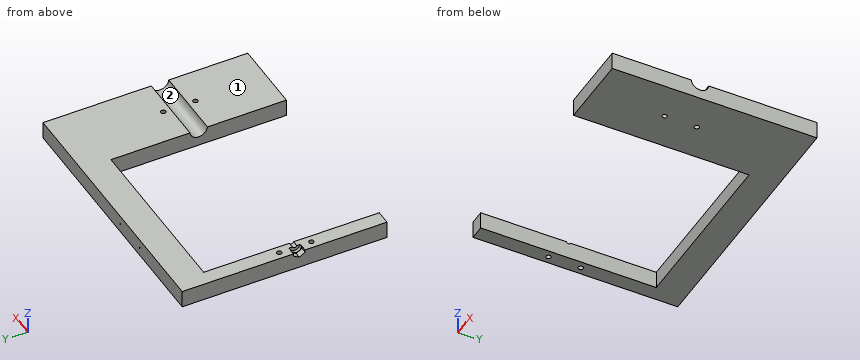
```python
from build123d import *

# Parameters (mm, degrees)
F0_W      = 180
F0_H      = 140
F1_DEPTH  = 30
F4_DEPTH  = 30
F5_DEPTH  = 4
F6_R      = 3.8
F7_DEPTH  = 2
F8_R      = 1.55
F9_DEPTH  = 7
F10_R     = 6
F12_DEPTH = 50
F11_R     = 0.5
F13_DEPTH = 1
F14_W     = 180
F14_H     = 140
F15_DEPTH = 18
F16_R     = 1.65
F17_DEPTH = 12


# Not quite as in the source:
# - a feature names something its author has since deleted; it is built from what else it names


with BuildPart() as f1:
    # F0 (on Top) → F1 (new body)
    with BuildSketch(Plane.XY):
        Rectangle(F0_W, F0_H)
    extrude(amount=F1_DEPTH)

    # F3 (on Top) → F4 (cut, through all)
    with BuildSketch(Plane.XY):
        Polygon((40, -70), (40, 0), (40, 50), (0, 50), (-80, 50), (-80, -70), align=None)
    extrude(amount=F4_DEPTH, mode=Mode.SUBTRACT)

    # F2 (on face) → F5 (cut)
    with BuildSketch(Plane(origin=(-90, 0, 0), x_dir=(0, -1, 0), z_dir=(-1, 0, 0))):
        Polygon((10, 17.12), (5.9989626345, 14.81), (5.9989626345, 10.19), (10, 7.88), (14.0010373655, 10.19), (14.0010373655, 14.81), align=None)
    extrude(amount=-F5_DEPTH, mode=Mode.SUBTRACT)

    # F6 (on face) → F7 (cut)
    with BuildSketch(Plane(origin=(-86, 0, 0), x_dir=(0, -1, 0), z_dir=(-1, 0, 0))):
        with Locations((10, 12.5)):
            Circle(F6_R)
    extrude(amount=-F7_DEPTH, mode=Mode.SUBTRACT)

    # F8 (on face) → F9 (cut)
    with BuildSketch(Plane(origin=(-84, 0, 0), x_dir=(0, -1, 0), z_dir=(-1, 0, 0))):
        with Locations((10, 12.5)):
            Circle(F8_R)
    extrude(amount=-F9_DEPTH, mode=Mode.SUBTRACT)

    # F10 (on face) → F12 (cut, through all)
    with BuildSketch(Plane.YZ.offset(90)):
        with Locations((-10, 12.5)):
            Circle(F10_R)
    extrude(amount=-F12_DEPTH, mode=Mode.SUBTRACT)

    # F11 (on face) → F13 (cut)
    with BuildSketch(Plane(origin=(0, 70, 0), x_dir=(-1, 0, 0), z_dir=(0, 1, 0))):
        with Locations((35, 6)):
            Circle(F11_R)
        with Locations((10, 6)):
            Circle(F11_R)
    extrude(amount=-F13_DEPTH, mode=Mode.SUBTRACT)

    # F14 (on face) → F15 (cut)
    with BuildSketch(Plane.XY.offset(30)):
        Rectangle(F14_W, F14_H)
    extrude(amount=-F15_DEPTH, mode=Mode.SUBTRACT)

    # F16 (on face) → F17 (cut, through all)
    with BuildSketch(Plane.XY.offset(12)):
        with Locations((65, 1)):
            Circle(F16_R)
        with Locations((65, -21)):
            Circle(F16_R)
        with Locations((-85, 1)):
            Circle(F16_R)
        with Locations((-85, -21)):
            Circle(F16_R)
    extrude(amount=-F17_DEPTH, mode=Mode.SUBTRACT)


solid = f1.part
```
Verification items for the finished model (mm, model axes). Face numbers are marked on the shaded views. Coordinates: 2 decimals unless noted, no trailing zeros. Write each loop counter-clockwise with the first axis right and the second up, starting at its lowest first coordinate (ties: lowest second). Pieces come first, ordered by that corner, then holes. Notation, with made-up numbers: (33, -1) - (45, -1) arc R20 cw to (45, 10) - close; hole circle Ø7 at (-4, 21.25). An arc over 180 degrees is marked (long way). Write item = value, one per line.
Q1. Cross-section at A-A (y = -56.5). Enter the section's corners in (x, z), plus the area to 3 significant figures.
Answer:
outline = (-90, 0) - (-80, 0) - (-80, 12) - (-90, 12) - close; (40, 0) - (90, 0) - (90, 12) - (40, 12) - close
area = 720 mm²
Q2. Mould release check, pull along Y, two halves, no side actions. Record for the marked faces 1 and 2: released by +Y, released by -Y, zero draft, split by the parting line, or undercut.
Answer:
face_1 = zero draft
face_2 = undercut
Q3. Cross-section at B-B (z = 2). Enter the section's corners in (x, y).
Answer:
outline = (-90, -70) - (-80, -70) - (-80, 50) - (40, 50) - (40, -70) - (90, -70) - (90, 70) - (-90, 70) - close; hole circle Ø3.3 at (-85, -21); hole circle Ø3.3 at (-85, 1); hole circle Ø3.3 at (65, -21); hole circle Ø3.3 at (65, 1)
Q4. Material ranges on L1, parallel to Y at x = 65, z = 5.75; L2, parallel to Z at x = -35, y = 69.4; L3, parallel to X at y = -17, z = 5, recorded low to high. Write a range as from..to.
Answer:
L1 = -70..-22.65, -19.35..-0.65, 2.65..70
L2 = 0..5.5, 6.5..12
L3 = -90..-80, 40..90
Q5. Go/stop test with flat-tipped pins: pin 1 Ø4.5 at (x, y) = (65, -21) entering from +Z; pin 2 Ø2.5 at (x, y) = (-85, -21) entering from -Z; pin 3 Ø3 at (x, z) = (-26.5, 3) entering from -Y; pin 4 Ø1.2 at (y, z) = (-10.5, 9) entering from -X. Record where each tip stops, or that it passes through.
Answer:
pin_1 = 12
pin_2 = through
pin_3 = 50
pin_4 = -86
Q6. Cross-section at C-C (x = 28). Enter the section's corners in (y, z), plus the area to 3 significant figures.
Answer:
outline = (50, 0) - (70, 0) - (70, 12) - (50, 12) - close
area = 240 mm²
